For this review, use the dimensioned drawing (mm, ordinates from the lowest corner) and the shaded views. Coordinates: 2 decimals unless noted, no trailing zeros. Loops run counter-clockwise (first coordinate to the right, second up) from the corner with the lowest first, then second, coordinate; pieces in that order, holes last. Notation, with made-up numbers: (12, 14) - (44, 14) arc R5 cw to (44, 23) - close; hole circle Ø6 at (19, 50.5). An arc over 180 degrees is marked (long way). Use a Markdown table: item, result. Add a question column.
1) Add section B-B, the plane x = 5. Give the boundary of the cut face in (y, z), and give its area (3 significant figures).
2) To check wall thickness, follow L1, parallel to X at y = 0.9, z = 47; L2, parallel to Z at x = 60, y = 0.5; L3, parallel to Z at x = 60, y = 1.2. State the ranges of each line that lie inside material, in increasing order. Write a range as [from, to].
3) Add section C-C, the plane y = 1.3. Give the boundary of the cut face in (x, z), and give its area (3 significant figures).
4) Add section A-A, the plane z = 47. Give the boundary of the cut face in (x, y).
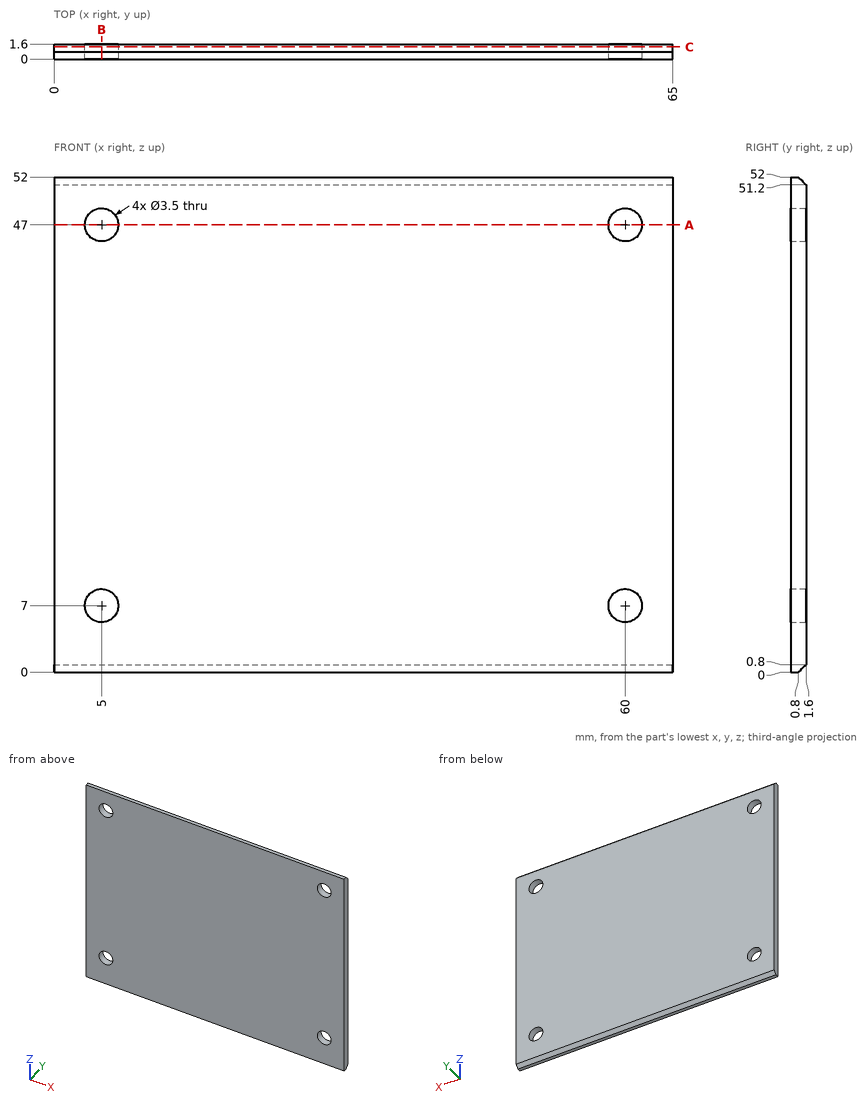
From the geometry:
| question | item | result |
|---|---|---|
| 1 | outline | (0, 0) - (0.8, 0) - (1.6, 0.8) - (1.6, 5.25) - (0, 5.25) - close; (0, 8.75) - (1.6, 8.75) - (1.6, 45.25) - (0, 45.25) - close; (0, 48.75) - (1.6, 48.75) - (1.6, 51.2) - (0.8, 52) - (0, 52) - close |
| 1 | area | 71.4 mm^2 |
| 2 | L1 | x = [0, 3.25], [6.75, 58.25], [61.75, 65] |
| 2 | L2 | z = [0, 5.25], [8.75, 45.25], [48.75, 52] |
| 2 | L3 | z = [0.4, 5.25], [8.75, 45.25], [48.75, 51.6] |
| 3 | outline | (0, 0.5) - (65, 0.5) - (65, 51.5) - (0, 51.5) - close; hole circle Ø3.5 at (5, 7); hole circle Ø3.5 at (5, 47); hole circle Ø3.5 at (60, 7); hole circle Ø3.5 at (60, 47) |
| 3 | area | 3,280 mm^2 |
| 4 | outline | (0, 0) - (3.25, 0) - (3.25, 1.6) - (0, 1.6) - close; (6.75, 0) - (58.25, 0) - (58.25, 1.6) - (6.75, 1.6) - close; (61.75, 0) - (65, 0) - (65, 1.6) - (61.75, 1.6) - close |
